Check sheet for the drawn part. Datum: minimum x, y, z corner. Units: mm. A direction names the side the tool comes from. Coordinates: 2 decimals unless noted, no trailing zeros. Loops run counter-clockwise (first coordinate to the right, second up) from the corner with the lowest first, then second, coordinate; pieces in that order, holes last.
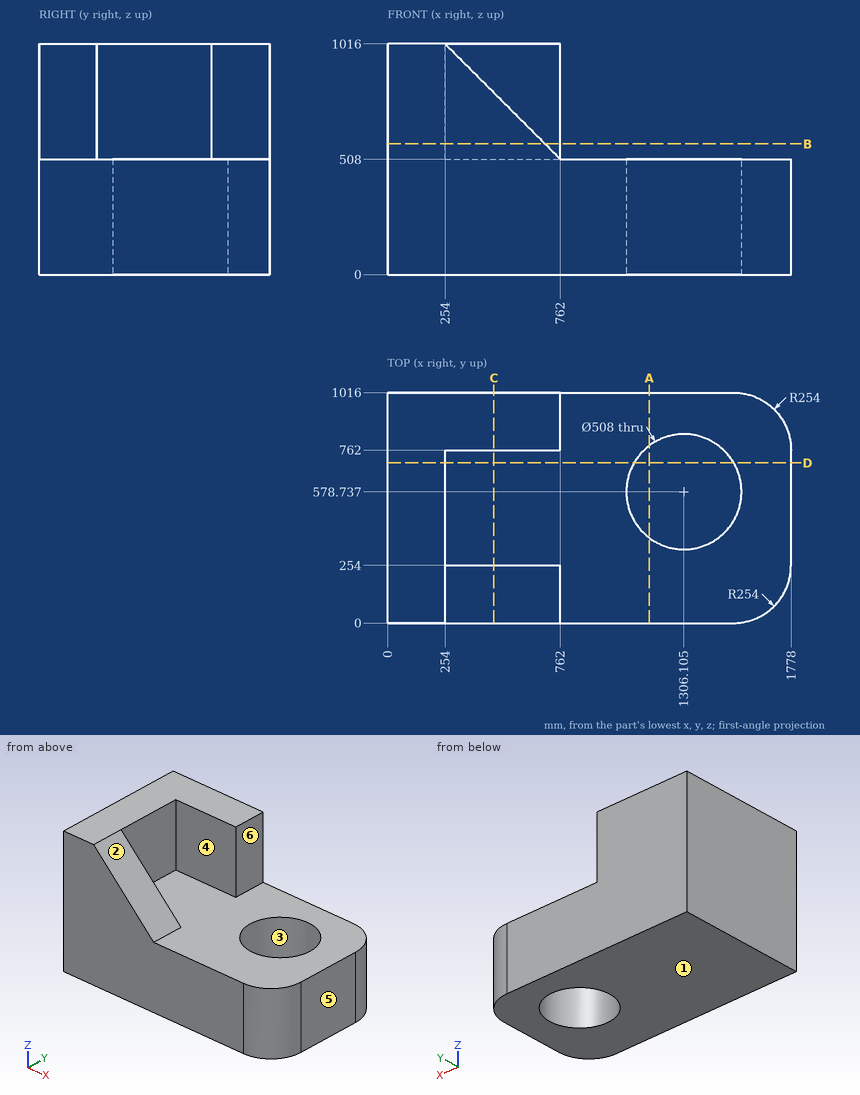
(1) Gauge pin test, flat ends, axial feed: pin 1 Ø8 at (y, z) = (869.5, 515.5) entering from +X; pin 2 Ø3 at (x, y) = (311, 905.5) entering from -Z. Record the tip position at first contact, or that the pin passes through.
Findings:
pin 1: stops at x = 762
pin 2: stops at z = 0
(2) Draft check along X on the marked faces 1, 2 and 3. Enter one of: +X half, -X half, draft (parallel to the pull), parting line (faces both ways), or undercut.
Findings:
face 1: draft
face 2: +X half
face 3: undercut
(3) Access from +Z, -Z, +X, -X, +Y, -Y to the whole of each face (thin tool, end or side, straight path). Record for the marked faces 4, 5 and 6.
Findings:
face 4: +Z, +X
face 5: +Z, -Z, +X, +Y, -Y
face 6: +Z, +X, +Y, -Y
(4) Sectioned sample at C-C on x = 468.5. Record the cut outline in (y, z), and give its area (3 significant figures).
Findings:
outline: (0, 0) - (1016, 0) - (1016, 1016) - (762, 1016) - (762, 508) - (254, 508) - (254, 801.5) - (0, 801.5) - close
area: 720,000 mm2
(5) Sectioned sample at D-D on y = 706.5. Record the cut outline in (x, z), and give its area (3 significant figures).
Findings:
outline: (0, 0) - (1086.58, 0) - (1086.58, 508) - (254, 508) - (254, 1016) - (0, 1016) - close; (1525.63, 0) - (1778, 0) - (1778, 508) - (1525.63, 508) - close
area: 809,000 mm2
(6) Scan lines: L1, parallel to Y at x = 473.5, z = 903; L2, parallel to X at y = 520, z = 660; L3, parallel to Z at x = 884, y = 807. Record each from-to range of solid material in increasing order.
Findings:
L1: y = 762 to 1016
L2: x = 0 to 254
L3: z = 0 to 508
(7) Sectioned sample at B-B on z = 575.5. Record the cut outline in (x, y).
Findings:
outline: (0, 0) - (694.5, 0) - (694.5, 254) - (254, 254) - (254, 762) - (762, 762) - (762, 1016) - (0, 1016) - close
(8) Sectioned sample at A-A on x = 1153.5. Record the cut outline in (y, z), and give its area (3 significant figures).
Findings:
outline: (0, 0) - (375.69, 0) - (375.69, 508) - (0, 508) - close; (781.78, 0) - (1016, 0) - (1016, 508) - (781.78, 508) - close
area: 310,000 mm2
